from build123d import *

# Parameters (mm, degrees)
SKETCH1_W           = 101.6
SKETCH1_H           = 88.9
BOSS_EXTRUDE1_DEPTH = 3.175
CUT_EXTRUDE1_DEPTH  = 68.576054376


with BuildPart() as part:
    # Sketch1 → Boss-Extrude1 (new body)
    with BuildSketch(Plane(origin=(0, 0, 0), x_dir=(1, 0, 0), z_dir=(0, 1, 0))):
        Rectangle(SKETCH1_W, SKETCH1_H)
    extrude(amount=BOSS_EXTRUDE1_DEPTH)

    # Sketch2 → Cut-Extrude1 (cut, through all)
    with BuildSketch(Plane(origin=(0, 3.175, 0), x_dir=(1, 0, 0), z_dir=(0, 1, 0))):
        with BuildLine():
            Line((-35.8, 39.564), (-30.8, 39.564))
            ThreePointArc((-30.8, 39.564), (-27.05, 35.814), (-30.8, 32.064))
            Line((-30.8, 32.064), (-35.8, 32.064))
            ThreePointArc((-35.8, 32.064), (-39.55, 35.814), (-35.8, 39.564))
        make_face()
        with BuildLine():
            Line((-35.8, -32.064), (-30.8, -32.064))
            ThreePointArc((-30.8, -32.064), (-27.05, -35.814), (-30.8, -39.564))
            Line((-30.8, -39.564), (-35.8, -39.564))
            ThreePointArc((-35.8, -39.564), (-39.55, -35.814), (-35.8, -32.064))
        make_face()
        with BuildLine():
            Line((3.5, 36.5), (6.5, 36.5))
            ThreePointArc((6.5, 36.5), (8, 35), (6.5, 33.5))
            Line((6.5, 33.5), (3.5, 33.5))
            ThreePointArc((3.5, 33.5), (2, 35), (3.5, 36.5))
        make_face()
        with BuildLine():
            Line((33.5, 36.5), (36.5, 36.5))
            ThreePointArc((36.5, 36.5), (38, 35), (36.5, 33.5))
            Line((36.5, 33.5), (33.5, 33.5))
            ThreePointArc((33.5, 33.5), (32, 35), (33.5, 36.5))
        make_face()
        with BuildLine():
            Line((3.5, -33.5), (6.5, -33.5))
            ThreePointArc((6.5, -33.5), (8, -35), (6.5, -36.5))
            Line((6.5, -36.5), (3.5, -36.5))
            ThreePointArc((3.5, -36.5), (2, -35), (3.5, -33.5))
        make_face()
        with BuildLine():
            Line((33.5, -33.5), (36.5, -33.5))
            ThreePointArc((36.5, -33.5), (38, -35), (36.5, -36.5))
            Line((36.5, -36.5), (33.5, -36.5))
            ThreePointArc((33.5, -36.5), (32, -35), (33.5, -33.5))
        make_face()
    extrude(amount=-CUT_EXTRUDE1_DEPTH, mode=Mode.SUBTRACT)


solid = part.part
Input: part model. Units: mm. Frame: model coordinates. Give positions to 0.01 mm unless a question says otherwise; leave off trailing zeros. Write each loop counter-clockwise with the first axis right and the second up, starting at its lowest first coordinate (ties: lowest second). Pieces come first, ordered by that corner, then holes.
Q1. Section B-B, the plane z = 35. Output: boundary loops of the cut face in (x, y) (3 decimals), plus the area to 3 significant figures.
Q2. Pull-direction query (Z, two-part tool) for faces 1 (the face through (-1, 2, 44.45)), 2 (the face through (-1, 0, -1)), 3 (the face through (5, 2, -33.5)); classes: pulls with the +Z half, pulls with the -Z half, needs draft (parallel to the pull), parting line crosses it, or undercut.
Q3. Section A-A, the plane y = 1.45. Output: boundary loops of the cut face in (x, z).
Q4. Material intervals for probe 1 along Z at (x, y) = (-32, 1); probe 2 along Z at (x, y) = (37, 1.2); probe 3 along X at (y, z) = (2.1, 39), sorted ascending.
Filled in:
1. outline: (-50.8, 0) - (-39.461, 0) - (-39.461, 3.175) - (-50.8, 3.175) - close; (-27.139, 0) - (2, 0) - (2, 3.175) - (-27.139, 3.175) - close; (8, 0) - (32, 0) - (32, 3.175) - (8, 3.175) - close; (38, 0) - (50.8, 0) - (50.8, 3.175) - (38, 3.175) - close
1. area: 245 mm2
2. face 1: pulls with the +Z half
2. face 2: needs draft
2. face 3: undercut
3. outline: (-50.8, -44.45) - (50.8, -44.45) - (50.8, 44.45) - (-50.8, 44.45) - close; hole (-35.8, -39.56) - (-30.8, -39.56) arc R3.75 ccw to (-30.8, -32.06) - (-35.8, -32.06) arc R3.75 ccw to start; hole (-35.8, 32.06) - (-30.8, 32.06) arc R3.75 ccw to (-30.8, 39.56) - (-35.8, 39.56) arc R3.75 ccw to start; hole (3.5, -36.5) - (6.5, -36.5) arc R1.5 ccw to (6.5, -33.5) - (3.5, -33.5) arc R1.5 ccw to start; hole (3.5, 33.5) - (6.5, 33.5) arc R1.5 ccw to (6.5, 36.5) - (3.5, 36.5) arc R1.5 ccw to start; hole (33.5, -36.5) - (36.5, -36.5) arc R1.5 ccw to (36.5, -33.5) - (33.5, -33.5) arc R1.5 ccw to start; hole (33.5, 33.5) - (36.5, 33.5) arc R1.5 ccw to (36.5, 36.5) - (33.5, 36.5) arc R1.5 ccw to start
4. probe 1: z = -44.45 to -39.56, -32.06 to 32.06, 39.56 to 44.45
4. probe 2: z = -44.45 to -36.41, -33.59 to 33.59, 36.41 to 44.45
4. probe 3: x = -50.8 to -37.78, -28.82 to 50.8
